Input: part model. Units: mm. Frame: model coordinates. A direction names the side the tool comes from. Coordinates: 2 decimals unless noted, no trailing zeros. Order: outer loops, then holes, each group sorted by start corner. A loop starts at its lowest first (then second) coordinate and runs counter-clockwise, first axis right, second up. Notation, with made-up numbers: (76.5, 14) -> (130.5, 14) arc R31 ccw to (130.5, 49) -> close; hole circle Ø2 at (-1.75, 69). An arc over 180 degrees is marked (long way). One line per question, with ' | ' between items.
```python
from build123d import *

# Parameters (mm, degrees)
SKETCH1_W                 = 82.55
SKETCH1_H                 = 72.39
BOSS_EXTRUDE1_DEPTH       = 16.51
SKETCH3_W                 = 76.708
SKETCH3_H                 = 66.548
CUT_EXTRUDE1_DEPTH        = 4.699
F_4_CLEARANCE_HOLE1_D     = 3.4544
F_4_CLEARANCE_HOLE1_DEPTH = 10.16
F_4_CLEARANCE_HOLE1_TIP   = 1.037806461
CUT_EXTRUDE2_DEPTH        = 8.255
CUT_EXTRUDE2_DEPTH_BACK   = 3.175
SKETCH9_W                 = 73.153706622
SKETCH9_H                 = 53.34
CUT_EXTRUDE3_DEPTH        = 8.382
SKETCH12_W                = 10.829569732
SKETCH12_H                = 12.611774214
SKETCH12_W_2              = 17.214227743
SKETCH12_H_2              = 33.027302542
SKETCH12_W_3              = 31.75
SKETCH12_H_3              = 19.685
CUT_EXTRUDE8_DEPTH        = 4.699
FILLET1_R                 = 2.54


with BuildPart() as part:
    # Sketch1 → Boss-Extrude1 (new body)
    with BuildSketch(Plane(origin=(0, 0, 0), x_dir=(1, 0, 0), z_dir=(0, 1, 0))):
        Rectangle(SKETCH1_W, SKETCH1_H)
    extrude(amount=BOSS_EXTRUDE1_DEPTH)

    # Sketch3 → Cut-Extrude1 (cut)
    with BuildSketch(Plane(origin=(0, 16.51, 0), x_dir=(1, 0, 0), z_dir=(0, 1, 0))):
        Rectangle(SKETCH3_W, SKETCH3_H)
    extrude(amount=-CUT_EXTRUDE1_DEPTH, mode=Mode.SUBTRACT)

    # #4 Clearance Hole1
    with Locations(Plane(origin=(0, 11.811, 0), x_dir=(1, 0, 0), z_dir=(0, 1, 0))):
        with Locations((-34.925, 29.845), (34.29, 28.575), (34.29, -29.845), (-34.925, -29.845)):
            Hole(F_4_CLEARANCE_HOLE1_D / 2, depth=F_4_CLEARANCE_HOLE1_DEPTH)
            with Locations((0, 0, -(F_4_CLEARANCE_HOLE1_DEPTH + F_4_CLEARANCE_HOLE1_TIP / 2))):  # 118° drill point
                Cone(0, F_4_CLEARANCE_HOLE1_D / 2, F_4_CLEARANCE_HOLE1_TIP, mode=Mode.SUBTRACT)

    # Sketch8 → Cut-Extrude2 (cut, two sides: drawn at the far end of the back side and taken through both)
    with BuildSketch(Plane(origin=(0, 11.811, 0), x_dir=(1, 0, 0), z_dir=(0, 1, 0)).offset(-CUT_EXTRUDE2_DEPTH_BACK)):
        Polygon((38.249468146, -29.845), (36.269734073, -26.416), (32.310265927, -26.416), (30.330531854, -29.845), (32.310265927, -33.274), (36.269734073, -33.274), align=None)
        Polygon((-30.818884886, 29.845), (-32.871942443, 33.401), (-36.978057557, 33.401), (-39.031115114, 29.845), (-36.978057557, 26.289), (-32.871942443, 26.289), align=None)
        Polygon((38.249468146, 28.575), (36.269734073, 32.004), (32.310265927, 32.004), (30.330531854, 28.575), (32.310265927, 25.146), (36.269734073, 25.146), align=None)
        Polygon((-30.965531854, -29.845), (-32.945265927, -26.416), (-36.904734073, -26.416), (-38.884468146, -29.845), (-36.904734073, -33.274), (-32.945265927, -33.274), align=None)
    extrude(amount=CUT_EXTRUDE2_DEPTH + CUT_EXTRUDE2_DEPTH_BACK, mode=Mode.SUBTRACT)

    # Sketch9 → Cut-Extrude3 (cut)
    with BuildSketch(Plane(origin=(0, 11.811, 0), x_dir=(1, 0, 0), z_dir=(0, 1, 0))):
        with Locations((1.777146689, -0.675914663)):
            Rectangle(SKETCH9_W, SKETCH9_H)
    extrude(amount=-CUT_EXTRUDE3_DEPTH, mode=Mode.SUBTRACT)

    # Sketch12 → Cut-Extrude8 (cut)
    with BuildSketch(Plane(origin=(0, 16.51, 0), x_dir=(1, 0, 0), z_dir=(0, 1, 0))):
        with Locations((-35.860215134, 0)):
            Rectangle(SKETCH12_W, SKETCH12_H)
        with Locations((32.667886129, 1.587498929)):
            Rectangle(SKETCH12_W_2, SKETCH12_H_2)
        with Locations((-0.9525, 26.3525)):
            Rectangle(SKETCH12_W_3, SKETCH12_H_3)
    extrude(amount=-CUT_EXTRUDE8_DEPTH, mode=Mode.SUBTRACT)

    # Fillet1
    # the kernel refuses this fillet: 2.54 mm, written as the material it takes off along each edge
    with BuildSketch(Plane(origin=(38.735, 13.97, 33.655), x_dir=(0, 1, 0), z_dir=(0, 0, 1))) as fillet1_piece_1_section:
        Polygon((0, 0), (FILLET1_R, 0), (FILLET1_R, -FILLET1_R), (0, -FILLET1_R), align=None)
    fillet1_piece_1 = extrude(amount=FILLET1_R, mode=Mode.PRIVATE)
    fillet1_piece_1 = fillet1_piece_1 - Plane(origin=(38.735, 13.97, 33.655), x_dir=(-0.7071067811865475, -0.7071067811865475, 0), z_dir=(0, 0, 1)) * Sphere(FILLET1_R, mode=Mode.PRIVATE)
    add(fillet1_piece_1, mode=Mode.SUBTRACT)
    with BuildSketch(Plane(origin=(38.735, 13.97, -33.655), x_dir=(0, 1, 0), z_dir=(0, 0, -1))) as fillet1_piece_2_section:
        Polygon((0, 0), (FILLET1_R, 0), (FILLET1_R, FILLET1_R), (0, FILLET1_R), align=None)
    fillet1_piece_2 = extrude(amount=FILLET1_R, mode=Mode.PRIVATE)
    fillet1_piece_2 = fillet1_piece_2 - Plane(origin=(38.735, 13.97, -33.655), x_dir=(-0.7071067811865475, -0.7071067811865475, 0), z_dir=(0, 0, -1)) * Sphere(FILLET1_R, mode=Mode.PRIVATE)
    add(fillet1_piece_2, mode=Mode.SUBTRACT)
    with BuildSketch(Plane(origin=(-38.735, 13.97, 33.655), x_dir=(0, 0, 1), z_dir=(-1, 0, 0))) as fillet1_piece_3_section:
        Polygon((0, 0), (FILLET1_R, 0), (FILLET1_R, FILLET1_R), (0, FILLET1_R), align=None)
    fillet1_piece_3 = extrude(amount=FILLET1_R, mode=Mode.PRIVATE)
    fillet1_piece_3 = fillet1_piece_3 - Plane(origin=(-38.735, 13.97, 33.655), x_dir=(0, -0.7071067811865475, -0.7071067811865475), z_dir=(-1, 0, 0)) * Sphere(FILLET1_R, mode=Mode.PRIVATE)
    add(fillet1_piece_3, mode=Mode.SUBTRACT)
    with BuildSketch(Plane(origin=(-38.735, 13.97, -33.655), x_dir=(-1, 0, 0), z_dir=(0, 0, -1))) as fillet1_piece_4_section:
        Polygon((0, 0), (FILLET1_R, 0), (FILLET1_R, FILLET1_R), (0, FILLET1_R), align=None)
    fillet1_piece_4 = extrude(amount=FILLET1_R, mode=Mode.PRIVATE)
    fillet1_piece_4 = fillet1_piece_4 - Plane(origin=(-38.735, 13.97, -33.655), x_dir=(0.7071067811865475, -0.7071067811865475, 0), z_dir=(0, 0, -1)) * Sphere(FILLET1_R, mode=Mode.PRIVATE)
    add(fillet1_piece_4, mode=Mode.SUBTRACT)
    with BuildSketch(Plane(origin=(41.275, 16.51, 8.576152342), x_dir=(-1, 0, 0), z_dir=(0, 0, 1))) as fillet1_piece_5:
        with BuildLine():
            CenterArc((FILLET1_R, FILLET1_R), FILLET1_R, 180, 90)
            Line((0, FILLET1_R), (0, 0))
            Line((0, 0), (FILLET1_R, 0))
        make_face()
    extrude(amount=25.078847658, mode=Mode.SUBTRACT)
    with BuildSketch(Plane(origin=(8.5725, 16.51, -36.195), x_dir=(0, -1, 0), z_dir=(1, 0, 0))) as fillet1_piece_6:
        with BuildLine():
            CenterArc((FILLET1_R, -FILLET1_R), FILLET1_R, 90, 90)
            Line((0, -FILLET1_R), (0, 0))
            Line((0, 0), (FILLET1_R, 0))
        make_face()
    extrude(amount=30.1625, mode=Mode.SUBTRACT)
    with BuildSketch(Plane(origin=(-41.275, 16.51, 33.655), x_dir=(0, -1, 0), z_dir=(0, 0, -1)), Plane(origin=(-41.275, 16.51, 0.044112893), x_dir=(0, -1, 0), z_dir=(0, 0, -1))) as fillet1_piece_7:
        with BuildLine():
            CenterArc((FILLET1_R, -FILLET1_R), FILLET1_R, 90, 90)
            Line((0, -FILLET1_R), (0, 0))
            Line((0, 0), (FILLET1_R, 0))
        make_face()
    extrude(amount=33.699112893, mode=Mode.SUBTRACT)
    with BuildSketch(Plane(origin=(41.275, 16.51, -33.655), x_dir=(-1, 0, 0), z_dir=(0, 0, 1))) as fillet1_piece_8:
        with BuildLine():
            CenterArc((FILLET1_R, FILLET1_R), FILLET1_R, 180, 90)
            Line((0, FILLET1_R), (0, 0))
            Line((0, 0), (FILLET1_R, 0))
        make_face()
    extrude(amount=21.9038498, mode=Mode.SUBTRACT)
    with BuildSketch(Plane(origin=(-38.735, 16.51, -36.195), x_dir=(0, -1, 0), z_dir=(1, 0, 0))) as fillet1_piece_9:
        with BuildLine():
            CenterArc((FILLET1_R, -FILLET1_R), FILLET1_R, 90, 90)
            Line((0, -FILLET1_R), (0, 0))
            Line((0, 0), (FILLET1_R, 0))
        make_face()
    extrude(amount=28.2575, mode=Mode.SUBTRACT)
    with BuildSketch(Plane(origin=(38.735, 16.51, 36.195), x_dir=(0, -1, 0), z_dir=(-1, 0, 0))) as fillet1_piece_10:
        with BuildLine():
            CenterArc((FILLET1_R, -FILLET1_R), FILLET1_R, 90, 90)
            Line((0, -FILLET1_R), (0, 0))
            Line((0, 0), (FILLET1_R, 0))
        make_face()
    extrude(amount=77.47, mode=Mode.SUBTRACT)
    with BuildSketch(Plane(origin=(-41.275, -6.35, -36.195), x_dir=(1, 0, 0), z_dir=(0, 1, 0)), Plane(origin=(41.275, -6.35, 36.195), x_dir=(-1, 0, 0), z_dir=(0, 1, 0)), Plane(origin=(-41.275, -6.35, 36.195), x_dir=(0, 0, -1), z_dir=(0, 1, 0))) as fillet1_piece_11:
        with BuildLine():
            CenterArc((FILLET1_R, -FILLET1_R), FILLET1_R, 90, 90)
            Line((0, -FILLET1_R), (0, 0))
            Line((0, 0), (FILLET1_R, 0))
        make_face()
    extrude(amount=20.32, mode=Mode.SUBTRACT)
    with BuildSketch(Plane(origin=(41.275, -6.35, -36.195), x_dir=(-1, 0, 0), z_dir=(0, 1, 0))) as fillet1_piece_12:
        with BuildLine():
            CenterArc((FILLET1_R, FILLET1_R), FILLET1_R, 180, 90)
            Line((0, FILLET1_R), (0, 0))
            Line((0, 0), (FILLET1_R, 0))
        make_face()
    extrude(amount=20.32, mode=Mode.SUBTRACT)


solid = part.part
```
1. Ray query, line 1 (Z direction, x = -21, y = 7.5) (3 decimals); line 2 (X direction, y = 9.25, z = -11) (3 decimals); line 3 (Z direction, x = 34.29, y = 4.5) (3 decimals). Return the intervals inside material, ascending. Write a range as [from, to].
Recorded:
line 1: z = [-36.195, -25.994], [27.346, 36.195] | line 2: x = [-41.275, -34.8], [38.354, 41.275] | line 3: z = [-36.195, -30.302], [-26.848, -25.994], [27.346, 28.118], [31.572, 36.195]
2. Access query for faces 4 (the face through (1, 8, -25.994)), 5 (the face through (40, 11.811, -2)), 6 (the face through (-40.51, 6.89, -35.47)), 7 (the face through (14.922, 14, -35)). Directions: +Z, -Z, +X, -X, +Y, -Y. A direction counts if a zero-diameter tool reaches every point of the face in a straight line with its end or side. Return the directions, or none.
Recorded:
face 4: +Y | face 5: +X, +Y | face 6: -Z, -X, +Y, -Y | face 7: -Z, +Y
3. Cut plane B-B, the plane x = -8.5. Return loops of the section in (y, z) (3 decimals).
Recorded:
outline: (0, -36.195) -> (11.811, -36.195) -> (11.811, -25.994) -> (3.429, -25.994) -> (3.429, 27.346) -> (11.811, 27.346) -> (11.811, 33.274) -> (16.51, 33.274) -> (16.51, 33.655) arc R2.54 ccw to (13.97, 36.195) -> (0, 36.195) -> close
4. Mould query, pull axis Z, two halves, no side actions, for faces 1 (the face through (-35.146, 0.793, -30.048)), 2 (the face through (-40.551, 15.746, 20.172)), 3 (the face through (26.662, 15.746, -35.471)). Classes: released by +Z, released by -Z, zero draft, split by the parting line, or undercut.
Recorded:
face 1: undercut | face 2: zero draft | face 3: released by -Z
5. Cut plane C-C, the plane z = -13.5. Return loops of the section in (x, y) (3 decimals).
Recorded:
outline: (-41.275, 0) -> (41.275, 0) -> (41.275, 11.811) -> (38.354, 11.811) -> (38.354, 3.429) -> (-34.8, 3.429) -> (-34.8, 11.811) -> (-38.354, 11.811) -> (-38.354, 16.51) -> (-38.735, 16.51) arc R2.54 ccw to (-41.275, 13.97) -> close
6. Pin query (flat end, axial travel): pin 1 Ø4.5 at (x, z) = (-34.925, -29.845) entering from -Y; pin 2 Ø1 at (x, z) = (1.5, -24.5) entering from +Y; pin 3 Ø3 at (x, z) = (40.5, 4) entering from +Y; pin 4 Ø2 at (x, z) = (-35, -31) entering from +Y. Return the tip coordinate at first contact, or that it passes through.
Recorded:
pin 1: stops at y = 0 | pin 2: stops at y = 3.43 | pin 3: stops at y = 11.81 | pin 4: stops at y = 8.64
7. Cut plane D-D, the plane z = 16. Return loops of the section in (x, y) (3 decimals).
Recorded:
outline: (-41.275, 0) -> (41.275, 0) -> (41.275, 13.97) arc R2.54 ccw to (38.735, 16.51) -> (38.354, 16.51) -> (38.354, 3.429) -> (-34.8, 3.429) -> (-34.8, 11.811) -> (-38.354, 11.811) -> (-38.354, 16.51) -> (-38.735, 16.51) arc R2.54 ccw to (-41.275, 13.97) -> close
8. Cut plane A-A, the plane y = 6.25. Return loops of the section in (x, z) (3 decimals).
Recorded:
outline: (-41.275, -33.655) arc R2.54 ccw to (-38.735, -36.195) -> (38.735, -36.195) arc R2.54 ccw to (41.275, -33.655) -> (41.275, 33.655) arc R2.54 ccw to (38.735, 36.195) -> (-38.735, 36.195) arc R2.54 ccw to (-41.275, 33.655) -> close; hole circle Ø3.454 at (-34.925, -29.845); hole circle Ø3.454 at (-34.925, 29.845); hole (-34.8, -25.994) -> (38.354, -25.994) -> (38.354, 27.346) -> (-34.8, 27.346) -> close; hole circle Ø3.454 at (34.29, -28.575); hole circle Ø3.454 at (34.29, 29.845)
